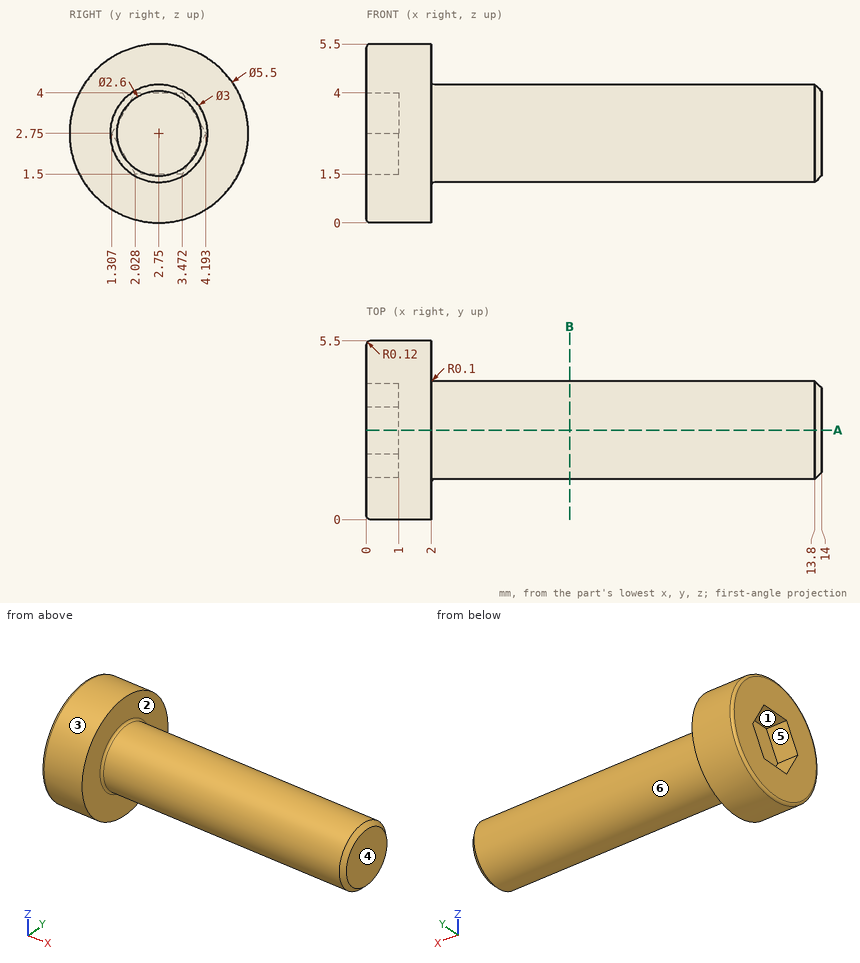
Could you check a few things on this drawing? It's one solid part, dimensions in mm from its lowest x, y, z. A direction names the side the tool comes from. Coordinates: 2 decimals unless noted, no trailing zeros. Loops run counter-clockwise (first coordinate to the right, second up) from the corner with the lowest first, then second, coordinate; pieces in that order, holes last.
1. We'd pull the mould along Y, two halves only. Please class the marked faces 1, 2 and 3: released by +Y, released by -Y, zero draft, split by the parting line, or undercut.
2. I need wall thicknesses on L1, parallel to X at y = 3.05, z = 3.5; L2, parallel to X at y = 4, z = 1.5; L3, parallel to Y at x = 8.25, z = 2.8. Which ranges of each line are inside material? Lowest first, please.
3. For the marked faces 4, 5 and 6, which set-ups out of +Z, -Z, +X, -X, +Y, -Y let a thin tool reach every point of the face, with its end or its side?
4. Imagine slicing it at A-A (y = 2.75). Please give me the cut outline in (x, z).
5. Imagine slicing it at B-B (x = 6.25). Please give me the cut outline in (y, z).
6. For P1, Ø3, axis at y = 3, z = 3, coming from the -X side; P2, Ø2, axis at x = 6, z = 4, coming from the +Y side; P3, Ø3, axis at x = 8, y = 4.5, coming from the +Z side; P4, Ø3, axis at y = 1, z = 5, coming from the +X side, each with a flat end and sliding along its axis, tell me the tip position at first contact or that it passes through.
Computed values:
1. face 1: undercut
1. face 2: zero draft
1. face 3: split by the parting line
2. L1: x = 1 to 14
2. L2: x = 0 to 2
2. L3: y = 1.25 to 4.25
3. face 4: +Z, -Z, +X, +Y, -Y
3. face 5: -X
3. face 6: +X
4. outline: (0, 0.12) arc R0.12 ccw to (0.12, 0) - (2, 0) - (2, 1.15) arc R0.1 cw to (2.1, 1.25) - (13.8, 1.25) - (14, 1.45) - (14, 4.05) - (13.8, 4.25) - (2.1, 4.25) arc R0.1 cw to (2, 4.35) - (2, 5.5) - (0.12, 5.5) arc R0.12 ccw to (0, 5.38) - (0, 4) - (1, 4) - (1, 1.5) - (0, 1.5) - close
5. outline: circle Ø3 at (2.75, 2.75)
6. P1: stops at x = 0
6. P2: stops at y = 4.23
6. P3: stops at z = 4.23
6. P4: stops at x = 13.95
